Here's how the part is built. I have some questions about the finished solid (model axes, mm). Face numbers are marked on the shaded views. A direction names the side the tool comes from. Round coordinates to 2 decimals unless told otherwise and drop trailing zeros. Write each loop counter-clockwise with the first axis right and the second up, starting at its lowest first coordinate (ties: lowest second). Pieces come first, ordered by that corner, then holes. Notation, with made-up numbers: (-10, -2) -> (30, -2) arc R15 cw to (30, 3) -> close; hole circle Ø7 at (26, 79.5). An arc over 180 degrees is marked (long way). Answer in a Markdown table with one row per item.
from build123d import *

# Parameters (mm, degrees)
SKETCH1_R             = 38
BOSS_EXTRUDE1_DEPTH   = 5
BOSS_EXTRUDE2_DEPTH   = 15
F_4_CLEARANCE_HOLE1_D = 3.4544
FILLET1_R             = 10
CHAMFER1_SIZE         = 1


with BuildPart() as part:
    # Sketch1 → Boss-Extrude1 (new body)
    with BuildSketch(Plane(origin=(0, 0, 0), x_dir=(0, 0, -1), z_dir=(1, 0, 0))):
        with BuildLine():
            Line((-28, -46.5), (28, -46.5))
            Line((28, -46.5), (41.098345354, -21.752609249))
            ThreePointArc((41.098345354, -21.752609249), (0, 46.5), (-41.098345354, -21.752609249))
            Line((-41.098345354, -21.752609249), (-28, -46.5))
        make_face()
        Circle(SKETCH1_R, mode=Mode.SUBTRACT)
    extrude(amount=BOSS_EXTRUDE1_DEPTH)

    # Sketch2 → Boss-Extrude2 (add)
    with BuildSketch(Plane(origin=(5, 0, 0), x_dir=(0, 0, -1), z_dir=(1, 0, 0))):
        Polygon((-28, -46.5), (28, -46.5), (35.484768774, -32.358633857), (34.60093339, -31.890835808), (25, -43.5), (-25, -43.5), (-34.60093339, -31.890835808), (-35.484768774, -32.358633857), align=None)
    extrude(amount=BOSS_EXTRUDE2_DEPTH)

    # #4 Clearance Hole1 (through all)
    with Locations(Plane.ZY):
        with Locations((-29.69848481, -29.69848481), (-29.69848481, 29.69848481), (29.69848481, 29.69848481), (29.69848481, -29.69848481)):
            Hole(F_4_CLEARANCE_HOLE1_D / 2)

    # Fillet1
    fillet1_edges = [part.edges().sort_by_distance(p)[0] for p in [
        (20, -32.124734832, -35.042851082),
        (20, -32.124734832, 35.042851082),
    ]]
    fillet(fillet1_edges, radius=FILLET1_R)

    # Chamfer1
    chamfer1_edges = [part.edges().sort_by_distance(p)[0] for p in [
        (20, -46.5, 0),
    ]]
    chamfer(chamfer1_edges, length=CHAMFER1_SIZE)


solid = part.part
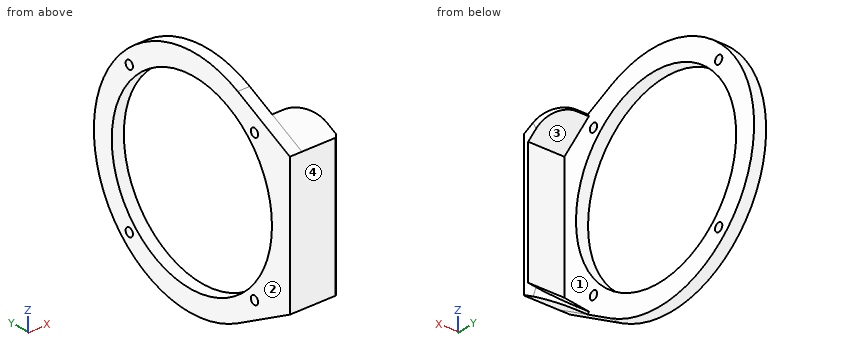
1) For pin 1 (4 mm diameter, centred on y = -36, z = -19.5, fed in from +X); pin 2 (4.5 mm diameter, centred on x = 10, z = 2, fed in from +Y); pin 3 (4 mm diameter, centred on x = 3.5, y = -2.5, fed in from +Z), each with a flat end and sliding along its axis, tell me the tip position at first contact or that it passes through.
Response:
| item | result |
|---|---|
| pin 1 | stops at x = 5 |
| pin 2 | stops at y = -43.5 |
| pin 3 | stops at z = 46.5 |
2) Which directions (+Z, -Z, +X, -X, +Y, -Y) give clear straight access to the entire face, cutting with the end or side of a thin tool? Please do the marked faces 3 and 4.
Response:
| item | result |
|---|---|
| face 3 | +X, +Y |
| face 4 | +Z, -Z, +X, -X, -Y |
3) I want a section at B-B, the plane y = 0. List the corners of the cut face in (x, z) for me.
Response:
| item | result |
|---|---|
| outline | (0, -46.5) -> (5, -46.5) -> (5, -38) -> (0, -38) -> close; (0, 38) -> (5, 38) -> (5, 46.5) -> (0, 46.5) -> close |
4) I want a section at A-A, the plane z = 0. List the corners of the cut face in (x, y) for me, and give its area (4 significant figures).
Response:
| item | result |
|---|---|
| outline | (0, -46.5) -> (19, -46.5) -> (20, -45.5) -> (20, -43.5) -> (5, -43.5) -> (5, -38) -> (0, -38) -> close; (0, 38) -> (5, 38) -> (5, 46.5) -> (0, 46.5) -> close |
| area | 129.5 mm^2 |
5) I need wall thicknesses on line 1 (Z direction, x = 4.5, y = 31); line 2 (Z direction, x = 4, y = 0.5); line 3 (Y direction, x = 7.75, z = -10). Which ranges of each line are inside material? Lowest first, please. Write a range as [from, to].
Response:
| item | result |
|---|---|
| line 1 | z = [-34.66, -30.83], [-28.56, -21.98], [21.98, 28.56], [30.83, 34.66] |
| line 2 | z = [-46.5, -38], [38, 46.5] |
| line 3 | y = [-46.5, -43.5] |
6) We'd pull the mould along Z, two halves only. Please class the marked faces 1 and 2: +Z half, -Z half, draft (parallel to the pull), parting line (faces both ways), or undercut.
Response:
| item | result |
|---|---|
| face 1 | undercut |
| face 2 | draft |
7) I want a section at D-D, the plane z = -12. List the corners of the cut face in (x, y) for me.
Response:
| item | result |
|---|---|
| outline | (0, -46.5) -> (19, -46.5) -> (20, -45.5) -> (20, -43.5) -> (5, -43.5) -> (5, -36.06) -> (0, -36.06) -> close; (0, 36.06) -> (5, 36.06) -> (5, 44.92) -> (0, 44.92) -> close |
8) I want a section at C-C, the plane x = 7.25. List the corners of the cut face in (y, z) for me, and give its area (3 significant figures).
Response:
| item | result |
|---|---|
| outline | (-46.5, -28) -> (-32.36, -35.48) -> (-31.89, -34.6) -> (-43.5, -25) -> (-43.5, 25) -> (-31.89, 34.6) -> (-32.36, 35.48) -> (-46.5, 28) -> close |
| area | 239 mm^2 |
